```python
from build123d import *

# Parameters (mm, degrees)
SKETCH2_R           = 2.75
SKETCH2_R_2         = 1.6
BOSS_EXTRUDE1_DEPTH = 2
FILLET1_R           = 1.5


with BuildPart() as part:
    # Sketch2 → Boss-Extrude1 (new body)
    with BuildSketch(Plane.XY):
        Polygon((-13.676428112, 164.5), (-83.975339533, 357.644671741), (-124.00010851, 357.644671741), (-53.701197089, 164.5), align=None)
        with Locations((-78.493044991, 250.157868697)):
            Circle(SKETCH2_R, mode=Mode.SUBTRACT)
        with Locations((-53.867594671, 182.5)):
            Circle(SKETCH2_R, mode=Mode.SUBTRACT)
        with Locations((-66.180319831, 216.328934348)):
            Circle(SKETCH2_R, mode=Mode.SUBTRACT)
        with Locations((-44.822322699, 172)):
            Circle(SKETCH2_R_2, mode=Mode.SUBTRACT)
        with Locations((-24.822322699, 172)):
            Circle(SKETCH2_R_2, mode=Mode.SUBTRACT)
        with Locations((-90.805770151, 283.986803045)):
            Circle(SKETCH2_R, mode=Mode.SUBTRACT)
        with Locations((-103.11849531, 317.815737393)):
            Circle(SKETCH2_R, mode=Mode.SUBTRACT)
        with Locations((-115.43122047, 351.644671741)):
            Circle(SKETCH2_R, mode=Mode.SUBTRACT)
        with Locations((-101.29954666, 351.411510234)):
            Circle(SKETCH2_R_2, mode=Mode.SUBTRACT)
    extrude(amount=BOSS_EXTRUDE1_DEPTH)

    # Fillet1
    fillet1_edges = [part.edges().sort_by_distance(p)[0] for p in [
        (-88.8506528, 261.072335871, 0),
        (-103.987724022, 357.644671741, 0),
        (-48.825883822, 261.072335871, 0),
        (-53.701197089, 164.5, 1),
        (-124.00010851, 357.644671741, 1),
        (-83.975339533, 357.644671741, 1),
    ]]
    fillet(fillet1_edges, radius=FILLET1_R)


solid = part.part
```
Read the model definition and answer for the solid it produces. Units are mm, in the model's axes. Give positions to 0.01 mm unless a question says otherwise; leave off trailing zeros. Answer in a Markdown table with one row per item.
1) This flat-tipped pin is pushed along its axis until it touches: pin 1 Ø5 at (x, y) = (-53.87, 182.5) entering from -Z. Where does it stop, or does it pass through?
Results list:
| item | result |
|---|---|
| pin 1 | through |
2) Section A-A on z = 1.1 is taken. Count the separate pieces of the cut face and the enclosed holes in it, plus the area to 3 significant figures.
Results list:
| item | result |
|---|---|
| separate pieces | 1 |
| enclosed holes | 9 |
| area | 7,540 mm^2 |
3) Straight lines are drawn through the part: line 1 (X direction, y = 184.5, z = 1.1); line 2 (X direction, y = 182.5, z = 0.6); line 3 (X direction, y = 239, z = 1.6). For each, find the intervals that lie inside material, in ascending order. Write a range as [from, to].
Results list:
| item | result |
|---|---|
| line 1 | [-60.92, -55.76], [-51.98, -21.01] |
| line 2 | [-59.93, -56.62], [-51.12, -20.55] |
| line 3 | [-80.82, -40.79] |
4) Determine the mould class of faces 1 (the cylindrical face through (-49.5, 261.8, 0.5)), 2 (the flat face through (-89.15, 261.89, 1.75)), 3 (the cylindrical face through (-89.537, 281.547, 0.986)) for opening direction Y: released by +Y, released by -Y, zero draft, split by the parting line, or undercut.
Results list:
| item | result |
|---|---|
| face 1 | released by +Y |
| face 2 | released by -Y |
| face 3 | undercut |
